Input: part model. Units: mm. Frame: model coordinates. Coordinates: 2 decimals unless noted, no trailing zeros. Order: outer loops, then holes, each group sorted by start corner. A loop starts at its lowest first (then second) coordinate and runs counter-clockwise, first axis right, second up. Notation, with made-up numbers: (-28.75, 71.25) -> (-1.75, 71.25) arc R23 ccw to (-1.75, 85.25) -> close; hole circle Ø10 at (-9.5, -33). An arc over 180 degrees is marked (long way). Use one line per item in the form item = value. Start each with the question number.
1) Section query B-B on y = 32. Output: boundary loops of the cut face in (x, z), then the cut area to 3 significant figures.
2) Section query A-A on z = 4.6. Output: boundary loops of the cut face in (x, y) (3 decimals), then the cut area to 3 significant figures.
3) Ray query, line 1 along Y through (x, z) = (10, 2.5); line 2 along Y through (x, z) = (194, 2.75); line 3 along Y through (x, z) = (38, 3.9) (3 decimals). Return the intervals inside material, ascending.
4) Pin query (flat end, axial travel): pin 1 (3.5 mm diameter, centred on x = -83, z = 2, fed in from -Y); pin 2 (5.5 mm diameter, centred on x = 156, y = -94, fed in from -Z); pin 3 (4.5 mm diameter, centred on x = -194, y = 88, fed in from +Z). Return the tip coordinate at first contact, or that it passes through.
from build123d import *

# Parameters (mm, degrees)
F1_DEPTH       = 3
F2_R           = 2
F3_DEPTH       = 3
F5_D           = 2.15
F5_DEPTH       = 3
F5_TIP         = 0.6459251655
F7_D           = 3.4
F7_CSINK_D     = 6.72
F7_CSINK_ANGLE = 90


with BuildPart() as f1:
    # F0 (on Top) → F1 (new body)
    with BuildSketch(Plane.XY):
        with BuildLine():
            Line((-130, 100), (-194, 100))
            ThreePointArc((-194, 100), (-198.2426406871, 98.2426406871), (-200, 94))
            Line((-200, 94), (-200, 0))
            Line((-200, 0), (-200, -94))
            ThreePointArc((-200, -94), (-198.2426406871, -98.2426406871), (-194, -100))
            Line((-194, -100), (-130, -100))
            Line((-130, -100), (-130, -75))
            Line((-130, -75), (-50, -75))
            Line((-50, -75), (-50, -100))
            Line((-50, -100), (70, -100))
            Line((70, -100), (70, -75))
            Line((70, -75), (150, -75))
            Line((150, -75), (150, -100))
            Line((150, -100), (165, -100))
            ThreePointArc((165, -100), (189.7487373415, -89.7487373415), (200, -65))
            Line((200, -65), (200, 0))
            Line((200, 0), (200, 65))
            ThreePointArc((200, 65), (189.7487373415, 89.7487373415), (165, 100))
            Line((165, 100), (150, 100))
            Line((150, 100), (150, 75))
            Line((150, 75), (70, 75))
            Line((70, 75), (70, 100))
            Line((70, 100), (-50, 100))
            Line((-50, 100), (-50, 75))
            Line((-50, 75), (-130, 75))
            Line((-130, 75), (-130, 100))
        make_face()
    extrude(amount=F1_DEPTH)

    # F2 (on face) → F3 (join)
    with BuildSketch(Plane.XY.offset(3)):
        with Locations((38, 42)):
            Circle(F2_R)
        with Locations((38, 65)):
            Circle(F2_R)
        with Locations((-20, 42)):
            Circle(F2_R)
        with Locations((-20, 65)):
            Circle(F2_R)
    extrude(amount=F3_DEPTH)

    # F5
    with Locations(Plane.XY.offset(6)):
        with Locations((-20, 42), (-20, 65), (38, 65), (38, 42)):
            Hole(F5_D / 2, depth=F5_DEPTH)
            with Locations((0, 0, -(F5_DEPTH + F5_TIP / 2))):  # 118° drill point
                Cone(0, F5_D / 2, F5_TIP, mode=Mode.SUBTRACT)

    # F7 (through all)
    with Locations(Plane(origin=(0, 0, 0), x_dir=(1, 0, 0), z_dir=(0, 0, -1))):
        with Locations((-136, -94), (-194, -88), (-194, 88), (-136, 94), (-44, 94), (10, 94), (64, 94), (156, 94), (194, 59), (194, 0), (194, -59), (156, -94), (64, -94), (10, -94), (-44, -94), (-194, 0)):
            CounterSinkHole(F7_D / 2, F7_CSINK_D / 2, counter_sink_angle=F7_CSINK_ANGLE)


solid = f1.part
Answers below:
q1.outline = (-200, 0) -> (200, 0) -> (200, 3) -> (-200, 3) -> close
q1.area = 1,200 mm^2
q2.outline = circle Ø4 at (-20, 42); circle Ø4 at (-20, 65); circle Ø4 at (38, 42); circle Ø4 at (38, 65); hole circle Ø2.15 at (-20, 42); hole circle Ø2.15 at (-20, 65); hole circle Ø2.15 at (38, 42); hole circle Ø2.15 at (38, 65)
q2.area = 35.7 mm^2
q3.line_1 = -100 to -95.7, -92.3 to 92.3, 95.7 to 100
q3.line_2 = -84.6 to -60.7, -57.3 to -1.7, 1.7 to 57.3, 60.7 to 84.6
q3.line_3 = 40 to 40.925, 43.075 to 44, 63 to 63.925, 66.075 to 67
q4.pin_1 = -75
q4.pin_2 = 0.61
q4.pin_3 = 3
